Read the model definition and answer for the solid it produces. Units are mm, in the model's axes. A direction names the side the tool comes from. Coordinates: 2 decimals unless noted, no trailing zeros. Order: outer loops, then holes, each group sorted by start corner. A loop starts at its lowest first (then second) coordinate and runs counter-clockwise, first axis right, second up.
```python
from build123d import *

# Parameters (mm, degrees)
SKETCH_1_W          = 50
SKETCH_1_H          = 150
EXTRUDE_1_DEPTH     = 25
CUT_EXTRUDE_1_DEPTH = 26
CHAMFER_1_SIZE      = 2


with BuildPart() as part:
    # Эскиз1 → Бобышка-Вытянуть1 (new body)
    with BuildSketch(Plane.XY):
        with Locations((25, 75)):
            Rectangle(SKETCH_1_W, SKETCH_1_H)
    extrude(amount=EXTRUDE_1_DEPTH)

    # Эскиз2 → Вырез-Вытянуть1 (cut, through all)
    with BuildSketch(Plane.XY.offset(25)):
        with BuildLine():
            Line((35.5, 125), (35.5, 25))
            ThreePointArc((35.5, 25), (25, 14.5), (14.5, 25))
            Line((14.5, 25), (14.5, 125))
            ThreePointArc((14.5, 125), (25, 135.5), (35.5, 125))
        make_face()
    extrude(amount=-CUT_EXTRUDE_1_DEPTH, mode=Mode.SUBTRACT)

    # Фаска1
    chamfer_1_edges = [part.edges().sort_by_distance(p)[0] for p in [
        (25, 14.5, 0),
        (14.5, 75, 0),
        (25, 135.5, 0),
        (35.5, 75, 0),
        (25, 14.5, 25),
        (35.5, 75, 25),
        (25, 135.5, 25),
        (14.5, 75, 25),
    ]]
    chamfer(chamfer_1_edges, length=CHAMFER_1_SIZE)


solid = part.part
```
1) A cutting plane is placed at C-C, the plane z = 6.25. Determine the outline of the cut face in (x, y).
A:
outline: (0, 0) - (50, 0) - (50, 150) - (0, 150) - close; hole (14.5, 25) arc R10.5 ccw to (35.5, 25) - (35.5, 125) arc R10.5 ccw to (14.5, 125) - close
2) Which of the six approach directions +Z, -Z, +X, -X, +Y, -Y give full straight-line access (tool end or side, diameter ignored) to faces 4 (the conical face through (25.2, 14.2, 23.3)), 5 (the flat face through (35.5, 76, 13)), 6 (the conical face through (25.2, 135.8, 1.7))?
A:
face 4: +Z
face 5: +Z, -Z
face 6: -Z
3) A cutting plane is placed at A-A, the plane y = 49. Determine the outline of the cut face in (x, z), and give its area (3 significant figures).
A:
outline: (0, 0) - (12.5, 0) - (14.5, 2) - (14.5, 23) - (12.5, 25) - (0, 25) - close; (35.5, 2) - (37.5, 0) - (50, 0) - (50, 25) - (37.5, 25) - (35.5, 23) - close
area: 717 mm2
4) Determine the mould class of faces 1 (the flat face through (50, 74, 12)), 2 (the flat face through (25, 150, 12)), 3 (the conical face through (24.8, 14.2, 1.7)) for opening direction Y: pulls with the +Y half, pulls with the -Y half, needs draft (parallel to the pull), parting line crosses it, or undercut.
A:
face 1: needs draft
face 2: pulls with the +Y half
face 3: undercut
5) A cutting plane is placed at B-B, the plane x = 25. Determine the outline of the cut face in (y, z), and give its area (3 significant figures).
A:
outline: (0, 0) - (12.5, 0) - (14.5, 2) - (14.5, 23) - (12.5, 25) - (0, 25) - close; (135.5, 2) - (137.5, 0) - (150, 0) - (150, 25) - (137.5, 25) - (135.5, 23) - close
area: 717 mm2
6) Straight lines are drawn through the part: line 1 (X direction, y = 67.5, z = 14); line 2 (X direction, y = 129, z = 22); line 3 (Y direction, x = 30, z = 9.25). For each, find the intervals that lie inside material, in ascending order.
A:
line 1: x = 0 to 14.5, 35.5 to 50
line 2: x = 0 to 15.29, 34.71 to 50
line 3: y = 0 to 15.77, 134.23 to 150
